from build123d import *

# Parameters (mm, degrees)
SKETCH1_R           = 3.81
BOSS_EXTRUDE1_DEPTH = 18.5775
BOSS_EXTRUDE2_START = 7.62
SKETCH2_R           = 10.9855
SKETCH2_R_2         = 3.81
BOSS_EXTRUDE2_DEPTH = 7.62
SKETCH3_R           = 6.35
CUT_EXTRUDE1_DEPTH  = 4.7625
CHAMFER1_SIZE       = 2.54
CHAMFER2_SIZE       = 0.762


with BuildPart() as part:
    # Sketch1 → Boss-Extrude1 (new body)
    with BuildSketch(Plane(origin=(0, 0, 0), x_dir=(0, 0, -1), z_dir=(1, 0, 0))):
        Polygon((3.592850725, 6.223), (-3.592850725, 6.223), (-7.18570145, 0), (-3.592850725, -6.223), (3.592850725, -6.223), (7.18570145, 0), align=None)
        Circle(SKETCH1_R, mode=Mode.SUBTRACT)
    extrude(amount=-BOSS_EXTRUDE1_DEPTH)

    # Sketch2 → Boss-Extrude2 (add)
    with BuildSketch(Plane(origin=(0, 0, 0), x_dir=(0, 0, -1), z_dir=(1, 0, 0)).offset(BOSS_EXTRUDE2_START)):
        with Locations(Location((0, 0, 0), (0, 0, 180))):
            Circle(SKETCH2_R)
        Circle(SKETCH2_R_2, mode=Mode.SUBTRACT)
    extrude(amount=-BOSS_EXTRUDE2_DEPTH)

    # Sketch3 → Cut-Extrude1 (cut)
    with BuildSketch(Plane(origin=(7.62, 0, 0), x_dir=(0, 0, -1), z_dir=(1, 0, 0))):
        Circle(SKETCH3_R)
    extrude(amount=-CUT_EXTRUDE1_DEPTH, mode=Mode.SUBTRACT)

    # Chamfer1
    chamfer1_edges = [part.edges().sort_by_distance(p)[0] for p in [
        (7.62, 0, -10.9855),
    ]]
    chamfer(chamfer1_edges, length=CHAMFER1_SIZE)

    # Chamfer2
    chamfer2_edges = [part.edges().sort_by_distance(p)[0] for p in [
        (2.8575, 0, 3.81),
        (-18.5775, 0, 3.81),
    ]]
    chamfer(chamfer2_edges, length=CHAMFER2_SIZE)


solid = part.part
Here's how the part is built. I have some questions about the finished solid (model axes, mm). A direction names the side the tool comes from. Coordinates: 2 decimals unless noted, no trailing zeros. Loops run counter-clockwise (first coordinate to the right, second up) from the corner with the lowest first, then second, coordinate; pieces in that order, holes last.
1. For P1, Ø2, axis at x = -16, z = -0.5, coming from the -Y side; P2, Ø5, axis at x = 3, y = -3, coming from the -Z side; P3, Ø6, axis at y = 0, z = 0, coming from the +X side; P4, Ø1, axis at x = -11.5, y = 5, coming from the +Z side, each with a flat end and sliding along its axis, tell me the tip position at first contact or that it passes through.
2. For faces 1 (the flat face through (-9.16, 3.16, 5.36)), 2 (the flat face through (-9.159, 3.068, -5.414)), 3 (the flat face through (-9, -6.223, 0)), 4 (the flat face through (-9.159, -3.068, 5.414)), 5 (the flat face through (0, 5, 5)), which set-ups out of +Z, -Z, +X, -X, +Y, -Y let a thin tool reach every point of the face, with its end or its side?
3. Imagine slicing it at B-B, the plane z = 0. Please give me the cut outline in (x, y).
4. I need wall thicknesses on L1, parallel to Y at x = 3.9, z = 0; L2, parallel to Y at x = -9.5, z = 0; L3, parallel to Z at x = -9.75, y = -1.5. Which ranges of each line are inside material? Lowest first, please.
5. Imagine slicing it at A-A, the plane x = -15.75. Please give me the cut outline in (y, z), and give its area (3 significant figures).
Taken from the geometry:
1. P1: stops at y = -6.22
1. P2: stops at z = -10.97
1. P3: passes through
1. P4: stops at z = 4.59
2. face 1: +Z, -X, +Y
2. face 2: -Z, -X, +Y
2. face 3: +Z, -Z, -X, -Y
2. face 4: +Z, -X, -Y
2. face 5: -X
3. outline: (-18.58, -6.22) - (0, -6.22) - (0, -10.99) - (5.08, -10.99) - (7.62, -8.45) - (7.62, -6.35) - (2.86, -6.35) - (2.86, -4.57) - (2.1, -3.81) - (-17.82, -3.81) - (-18.58, -4.57) - close; (-18.58, 4.57) - (-17.82, 3.81) - (2.1, 3.81) - (2.86, 4.57) - (2.86, 6.35) - (7.62, 6.35) - (7.62, 8.45) - (5.08, 10.99) - (0, 10.99) - (0, 6.22) - (-18.58, 6.22) - close
4. L1: y = -10.99 to -6.35, 6.35 to 10.99
4. L2: y = -6.22 to -3.81, 3.81 to 6.22
4. L3: z = -6.32 to -3.5, 3.5 to 6.32
5. outline: (-6.22, -3.59) - (0, -7.19) - (6.22, -3.59) - (6.22, 3.59) - (0, 7.19) - (-6.22, 3.59) - close; hole circle Ø7.62 at (0, 0)
5. area: 88.5 mm2
